The figure shows three views and two pictorial views of one solid part (mm, origin at its lowest corner). Answer the questions. Coordinates: 2 decimals unless noted, no trailing zeros. Loops run counter-clockwise (first coordinate to the right, second up) from the corner with the lowest first, then second, coordinate; pieces in that order, holes last. Notation, with made-up numbers: (9, -17.5) -> (53, -17.5) arc R31 cw to (53, 20.5) -> close; hole circle Ø7 at (42.25, -14). An arc over 180 degrees is marked (long way). Use a Markdown table: item, result. Add a question column.
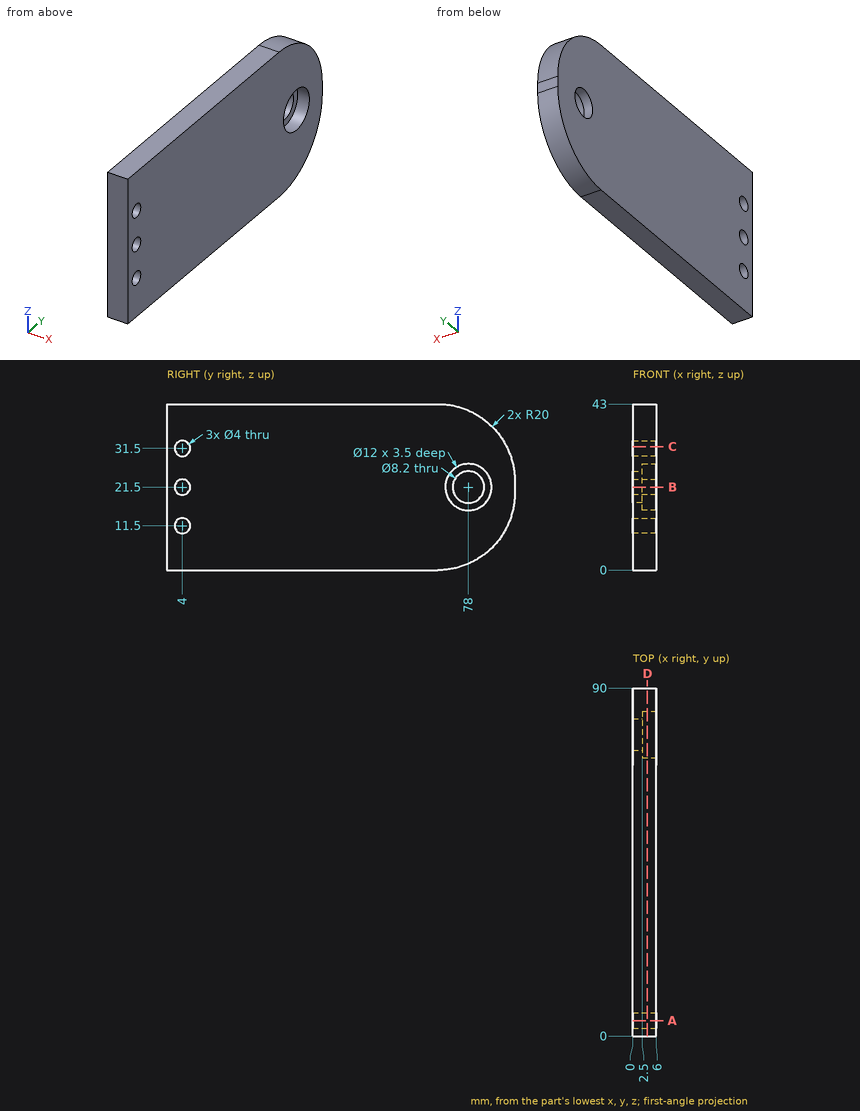
Item 1: Section A-A (y = 4) is taken. Determine the outline of the cut face in (x, z), then the cut area to 3 significant figures.
Item 2: Section D-D (x = 3.75) is taken. Determine the outline of the cut face in (y, z).
Item 3: Section B-B (z = 21.5) is taken. Determine the outline of the cut face in (x, y), then the cut area to 4 significant figures.
Item 4: Find the intervals of material crossed by probe 1 along Y at (x, z) = (4.1, 21.5); probe 2 along Y at (x, z) = (2, 21.5); probe 3 along X at (y, z) = (73.5, 22), in increasing order.
Item 5: Section C-C (z = 32) is taken. Determine the outline of the cut face in (x, y), then the cut area to 3 significant figures.
Output:
| question | item | result |
|---|---|---|
| 1 | outline | (0, 0) -> (6, 0) -> (6, 9.5) -> (0, 9.5) -> close; (0, 13.5) -> (6, 13.5) -> (6, 19.5) -> (0, 19.5) -> close; (0, 23.5) -> (6, 23.5) -> (6, 29.5) -> (0, 29.5) -> close; (0, 33.5) -> (6, 33.5) -> (6, 43) -> (0, 43) -> close |
| 1 | area | 186 mm2 |
| 2 | outline | (0, 0) -> (70, 0) arc R20 ccw to (90, 20) -> (90, 23) arc R20 ccw to (70, 43) -> (0, 43) -> close; hole circle Ø4 at (4, 11.5); hole circle Ø4 at (4, 21.5); hole circle Ø4 at (4, 31.5); hole circle Ø12 at (78, 21.5) |
| 3 | outline | (0, 0) -> (6, 0) -> (6, 2) -> (0, 2) -> close; (0, 6) -> (6, 6) -> (6, 72) -> (2.5, 72) -> (2.5, 73.9) -> (0, 73.9) -> close; (0, 82.1) -> (2.5, 82.1) -> (2.5, 84) -> (6, 84) -> (6, 90) -> (0, 90) -> close |
| 3 | area | 453.5 mm2 |
| 4 | probe 1 | y = 0 to 2, 6 to 72, 84 to 90 |
| 4 | probe 2 | y = 0 to 2, 6 to 73.9, 82.1 to 90 |
| 4 | probe 3 | x = 0 to 2.5 |
| 5 | outline | (0, 0) -> (6, 0) -> (6, 2.06) -> (0, 2.06) -> close; (0, 5.94) -> (6, 5.94) -> (6, 87.86) -> (0, 87.86) -> close |
| 5 | area | 504 mm2 |
